```python
from build123d import *

# Parameters (mm, degrees)
F0_R     = 56
F0_R_2   = 52.5
F1_DEPTH = 45
F2_R     = 56
F2_R_2   = 52.5
F2_R_3   = 48.5
F3_DEPTH = 10
F4_R     = 56
F4_R_2   = 52.5
F5_DEPTH = 45


with BuildPart() as f1:
    # F0 (on Front) → F1 (new body)
    with BuildSketch(Plane.XZ):
        Circle(F0_R)
        Circle(F0_R_2, mode=Mode.SUBTRACT)
    extrude(amount=F1_DEPTH)

    # F2 (on face) → F3 (join)
    with BuildSketch(Plane.XZ.offset(45)):
        Circle(F2_R)
        Circle(F2_R_2, mode=Mode.SUBTRACT)
        Circle(F2_R_2)
        Circle(F2_R_3, mode=Mode.SUBTRACT)
    extrude(amount=F3_DEPTH)

    # F4 (on face) → F5 (join)
    with BuildSketch(Plane.XZ.offset(55)):
        Circle(F4_R)
        Circle(F4_R_2, mode=Mode.SUBTRACT)
    extrude(amount=F5_DEPTH)


solid = f1.part
```
Here's how the part is built. I have some questions about the finished solid (model axes, mm). A direction names the side the tool comes from. Coordinates: 2 decimals unless noted, no trailing zeros. Order: outer loops, then holes, each group sorted by start corner. A loop starts at its lowest first (then second) coordinate and runs counter-clockwise, first axis right, second up. Notation, with made-up numbers: (50, 36) - (65, 36) arc R22 ccw to (65, 54) - close; hole circle Ø2 at (45.25, -2). An arc over 180 degrees is marked (long way). One line per question, with ' | ' between items.
(1) For faces 1 (the flat face through (-17, -100, 50)), 2 (the flat face through (15.3, -55, -46.4)), 3 (the cylindrical face through (50.076, -22.185, 15.77)), which set-ups out of +Z, -Z, +X, -X, +Y, -Y let a thin tool reach every point of the face, with its end or its side?
Report:
face 1: +Z, -Z, +X, -X, -Y | face 2: -Y | face 3: +Y
(2) Suppose I cut it at A-A on x = 0. List the corners of the cut face in (y, z) for me.
Report:
outline: (-100, -56) - (0, -56) - (0, -52.5) - (-45, -52.5) - (-45, -48.5) - (-55, -48.5) - (-55, -52.5) - (-100, -52.5) - close; (-100, 52.5) - (-55, 52.5) - (-55, 48.5) - (-45, 48.5) - (-45, 52.5) - (0, 52.5) - (0, 56) - (-100, 56) - close
(3) Will these pins go through, and if not, where does the flat tip stop? pin 1 (10 mm diameter, centred on x = 28, y = -65.5, fed in from +Z); pin 2 (6 mm diameter, centred on y = -55.5, z = -16, fed in from +X); pin 3 (1 mm diameter, centred on x = 39, y = -35, fed in from -Z).
Report:
pin 1: stops at z = 51.06 | pin 2: stops at x = 54.47 | pin 3: stops at z = -40.67
(4) Suppose I cut it at C-C on y = -23. List the corners of the cut face in (x, z) for me, and give its area (3 significant figures).
Report:
outline: circle Ø112 at (0, 0); hole circle Ø105 at (0, 0) | area: 1,190 mm2
(5) Suppose I cut it at B-B on z = 0. List the corners of the cut face in (x, y) for me, and give its area (3 significant figures).
Report:
outline: (-56, -100) - (-52.5, -100) - (-52.5, -55) - (-48.5, -55) - (-48.5, -45) - (-52.5, -45) - (-52.5, 0) - (-56, 0) - close; (48.5, -55) - (52.5, -55) - (52.5, -100) - (56, -100) - (56, 0) - (52.5, 0) - (52.5, -45) - (48.5, -45) - close | area: 780 mm2
(6) If we mould it in two halves opening along X, with no side actions, what happens to faces 4 (the cylindrical face through (22.38, -49.93, -43.028)), 5 (the cylindrical face through (51.73, -49.3, -21.45)), 6 (the flat face through (-17, 0, 50)), 7 (the flat face through (15.3, -45, -46.4))? For each: pulls with the +X half, pulls with the -X half, needs draft (parallel to the pull), parting line crosses it, or undercut.
Report:
face 4: undercut | face 5: parting line crosses it | face 6: needs draft | face 7: undercut
(7) If I drill on L1, parallel to Z at x = 0, y = -46.75; L2, parallel to Z at x = 0, y = -67.5; L3, parallel to X at y = -31.5, z = -37, over which ranges is the centre line in solid material (lowest first)?
Report:
L1: z = -56 to -48.5, 48.5 to 56 | L2: z = -56 to -52.5, 52.5 to 56 | L3: x = -42.04 to -37.25, 37.25 to 42.04
